Design review of the part built by this model. Coordinates are the model's own, in mm. A direction names the side the tool comes from. Give positions to 0.01 mm unless a question says otherwise; leave off trailing zeros. Loops run counter-clockwise (first coordinate to the right, second up) from the corner with the lowest first, then second, coordinate; pieces in that order, holes last. Notation, with made-up numbers: M 25,78 L 69,78 A13 cw 69,90 Z; hole C 18.5,86.5 d4. An arc over 180 degrees is marked long. Use a Markdown table: item, result. Add a question column.
(1) For probe 1 along Z at (x, y) = (98.75, 0); probe 2 along Y at (x, z) = (103, 52.5); probe 3 along Y at (x, z) = (100, 52), list the stretches that pass through material, from the lowest coordinate up.
(2) Insertion check: pin 1 Ø12 at (x, z) = (24, 76) entering from +Y; pin 2 Ø8 at (x, y) = (-17.5, 66.5) entering from -Z; pin 3 Ø3 at (x, y) = (57, 3.5) entering from +Z. Each pin has a flat end and moves straight along its axis. Give the tip position at first contact, or say it passes through.
(3) Draft analysis for pull direction Z (two halves, no side actions). For faces 5 (the face through (-1, 1, 0)), 6 (the face through (-91.771, 65, 50)), 7 (the face through (105, -1, 49)), state which applies: pulls with the +Z half, pulls with the -Z half, needs draft (parallel to the pull), parting line crosses it, or undercut.
(4) Add section B-B, the plane x = 75. Give the boundary of the cut face in (y, z), then the cut area to 3 significant figures.
(5) Add section A-A, the plane z = 52.5. Give the boundary of the cut face in (x, y).
(6) Add section D-D, the plane z = 68.5. Give the boundary of the cut face in (x, y), then the cut area to 3 significant figures.
(7) Add section C-C, the plane y = 0. Give the boundary of the cut face in (x, z), then the cut area to 3 significant figures.
(8) For faces 1 (the face through (100.07, 1.34, 54.61)), 2 (the face through (-95, -1, 54)), 3 (the face through (-1, -70, 94)), 4 (the face through (86.7, -64.9, 83.6)), list the 3-axis set-ups (+Z, -Z, +X, -X, +Y, -Y) from which the entire face can be reached by the end or side of a thin tool; tool diameter is ignored.
```python
from build123d import *

# Parameters (mm, degrees)
F1_DEPTH = 10
F0_W     = 210
F0_H     = 140
F2_DEPTH = 100
F3_W     = 180
F3_H     = 70
F4_DEPTH = 202.553704
F5_R     = 2.5
F6_DEPTH = 10
F7_R     = 5


with BuildPart() as f1:
    # F0 (on Top) → F1 (new body)
    with BuildSketch(Plane.XY):
        Polygon((82.656699, -60), (95, -60), (95, 60), (82.656699, 60), (72.656699, 60), (-95, 60), (-95, -60), (72.656699, -60), align=None)
    extrude(amount=F1_DEPTH)

    # F0 (on Top) → F2 (join)
    with BuildSketch(Plane.XY):
        Rectangle(F0_W, F0_H)
        Polygon((95, 60), (95, -60), (82.656699, -60), (72.656699, -60), (-95, -60), (-95, 60), (72.656699, 60), (82.656699, 60), align=None, mode=Mode.SUBTRACT)
    extrude(amount=F2_DEPTH)

    # F3 (on face) → F4 (cut)
    with BuildSketch(Plane.XZ.offset(70)):
        with Locations((-1.771243, 50)):
            Rectangle(F3_W, F3_H)
    extrude(amount=-F4_DEPTH, mode=Mode.SUBTRACT)

    # F5 (on face) → F6 (cut)
    with BuildSketch(Plane.YZ.offset(105)):
        with Locations((0, 52.499999)):
            Circle(F5_R)
    extrude(amount=-F6_DEPTH, mode=Mode.SUBTRACT)

    # F7
    f7_edges = [f1.edges().sort_by_distance(p)[0] for p in [
        (-91.771243, -65, 15),
        (-91.771243, 65, 15),
        (-91.771243, -65, 85),
        (-91.771243, 65, 85),
        (88.228757, -65, 15),
        (88.228757, 65, 15),
        (88.228757, -65, 85),
        (88.228757, 65, 85),
    ]]
    fillet(f7_edges, radius=F7_R)


solid = f1.part
```
Established:
| question | item | result |
|---|---|---|
| 1 | probe 1 | 0 to 50, 55 to 100 |
| 1 | probe 2 | -70 to -2.5, 2.5 to 70 |
| 1 | probe 3 | -70 to -2.45, 2.45 to 70 |
| 2 | pin 1 | through |
| 2 | pin 2 | z = 0 |
| 2 | pin 3 | z = 10 |
| 3 | face 5 | pulls with the -Z half |
| 3 | face 6 | undercut |
| 3 | face 7 | needs draft |
| 4 | outline | M -70,0 L 70,0 L 70,15 L 60,15 L 60,10 L -60,10 L -60,15 L -70,15 Z; M -70,85 L -60,85 L -60,100 L -70,100 Z; M 60,85 L 70,85 L 70,100 L 60,100 Z |
| 4 | area | 1,800 mm^2 |
| 5 | outline | M -105,-70 L -91.77,-70 L -91.77,-60 L -95,-60 L -95,60 L -91.77,60 L -91.77,70 L -105,70 Z; M 88.23,-70 L 105,-70 L 105,-2.5 L 95,-2.5 L 95,-60 L 88.23,-60 Z; M 88.23,60 L 95,60 L 95,2.5 L 105,2.5 L 105,70 L 88.23,70 Z |
| 6 | outline | M -105,-70 L -91.77,-70 L -91.77,-60 L -95,-60 L -95,60 L -91.77,60 L -91.77,70 L -105,70 Z; M 88.23,-70 L 105,-70 L 105,70 L 88.23,70 L 88.23,60 L 95,60 L 95,-60 L 88.23,-60 Z |
| 6 | area | 3,000 mm^2 |
| 7 | outline | M -105,0 L 105,0 L 105,50 L 95,50 L 95,10 L -95,10 L -95,100 L -105,100 Z; M 95,55 L 105,55 L 105,100 L 95,100 Z |
| 7 | area | 3,850 mm^2 |
| 8 | face 1 | +X |
| 8 | face 2 | +Z |
| 8 | face 3 | +Z, -Z, +X, -X, -Y |
| 8 | face 4 | +Y, -Y |
